Can you work these out from the drawing? Everything is in mm from the part's minimum corner. A direction names the side the tool comes from. Give positions to 0.01 mm unless a question says otherwise; leave off trailing zeros. Loops run counter-clockwise (first coordinate to the right, second up) from the corner with the lowest first, then second, coordinate; pieces in that order, holes last. Notation, with made-up numbers: (64, 57.25) -> (84, 57.25) arc R18 ccw to (84, 66.25) -> close; hole circle Ø7 at (73, 0.25). An arc over 180 degrees is marked (long way). Return JSON: item names as keys, results as strings. Group by question number.
Q1. Suppose I cut it at C-C, the plane z = 4.25. Please give me the cut outline in (x, y) (1 decimal).
Q2. Suppose I cut it at A-A, the plane y = 5. Please give me the cut outline in (x, z), and give its area (3 significant figures).
Q3. Which directions (+Z, -Z, +X, -X, +Y, -Y) give clear straight access to the entire face, cutting with the end or side of a thin tool? Please do the marked faces 4, 5 and 6.
Q4. Suppose I cut it at D-D, the plane y = 13.75. Please give me the cut outline in (x, z).
Q5. Suppose I cut it at B-B, the plane x = 3.25. Please give me the cut outline in (y, z).
Q6. Will these pins go through, and if not, where does the flat tip stop? pin 1 (5 mm diameter, centred on x = 5, y = 5, fed in from -Z); pin 2 (1 mm diameter, centred on y = 9, z = 7.5, fed in from -X); pin 3 (4.5 mm diameter, centred on y = 15.12, z = 5, fed in from +X); pin 4 (2 mm diameter, centred on y = 17, z = 5.5, fed in from -X).
Q7. I need wall thicknesses on line 1 along X through (y, z) = (5, 2); line 2 along Y through (x, z) = (3.75, 1.25) (1 decimal); line 3 along X through (y, z) = (1, 9.25). Which ranges of each line are inside material? Lowest first, please. Write a range as [from, to].
Q8. Thinking about a two-plate mould opening in Y: for the marked faces 1, 2 and 3, which applies, pulls with the +Y half, pulls with the -Y half, needs draft (parallel to the pull), parting line crosses it, or undercut?
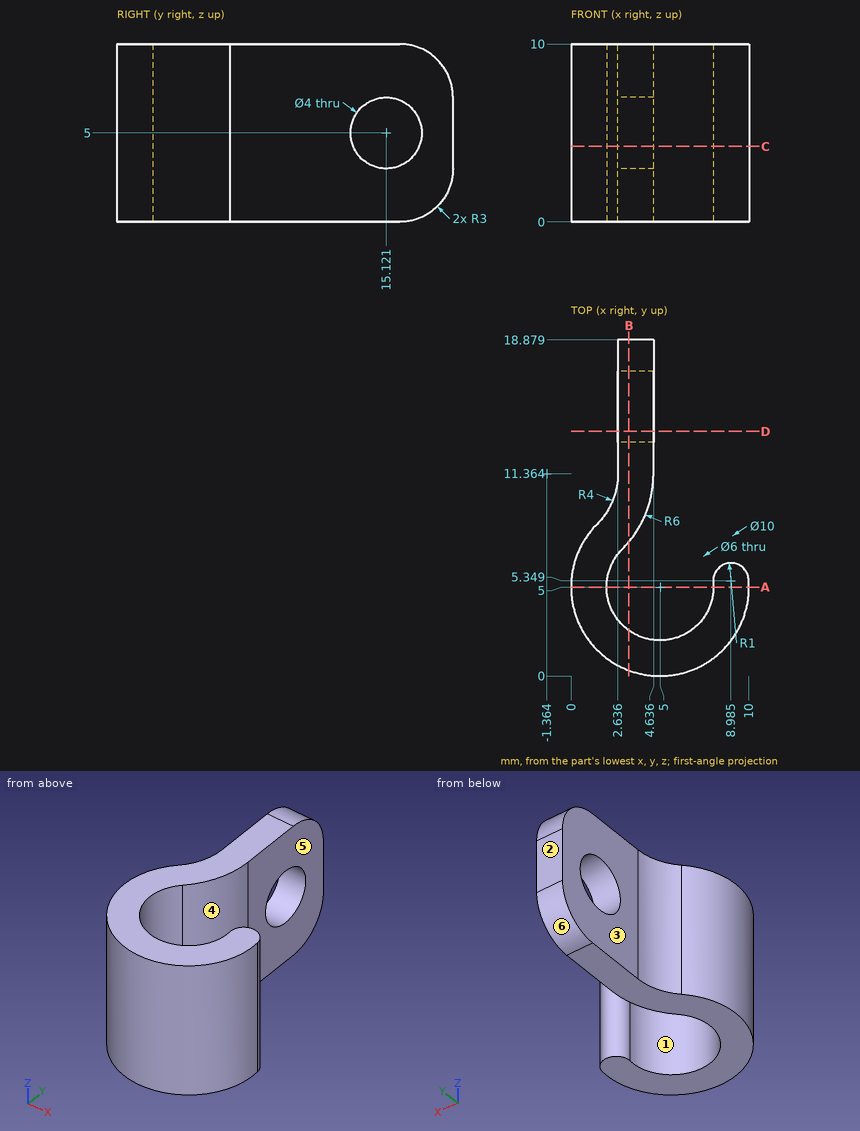
Ans:
{
 "1": {"outline": "(1.5, 8.5) arc R5 ccw (long way) to (10, 5.4) arc R1 ccw to (8, 5.3) arc R3 cw (long way) to (2.9, 7.1) arc R6 ccw to (4.6, 11.4) -> (4.6, 13.3) -> (2.6, 13.3) -> (2.6, 11.4) arc R4 cw to start; (2.6, 17) -> (4.6, 17) -> (4.6, 18.9) -> (2.6, 18.9) -> close"},
 "2": {"outline": "(0, 0) -> (2, 0) -> (2, 10) -> (0, 10) -> close; (8, 0) -> (10, 0) -> (10, 10) -> (8, 10) -> close", "area": "40.0 mm^2"},
 "3": {"face 4": "+Z, -Z, +X", "face 5": "+Z, -Z, +X, +Y", "face 6": "-Z, +X, -X, +Y"},
 "4": {"outline": "(2.64, 0) -> (4.64, 0) -> (4.64, 3.54) -> (2.64, 3.54) -> close; (2.64, 6.46) -> (4.64, 6.46) -> (4.64, 10) -> (2.64, 10) -> close"},
 "5": {"outline": "(0.32, 0) -> (2.56, 0) -> (2.56, 10) -> (0.32, 10) -> close; (7.53, 0) -> (15.88, 0) arc R3 ccw to (18.88, 3) -> (18.88, 7) arc R3 ccw to (15.88, 10) -> (7.53, 10) -> close; hole circle Ø4 at (15.12, 5)"},
 "6": {"pin 1": "passes through", "pin 2": "stops at x = 1.43", "pin 3": "stops at x = 4.64", "pin 4": "stops at x = 2.64"},
 "7": {"line 1": "x = [0, 2], [8, 10]", "line 2": "y = [0.2, 2.3], [8.2, 18.3]", "line 3": "x = [2, 8]"},
 "8": {"face 1": "undercut", "face 2": "pulls with the +Y half", "face 3": "needs draft"}
}
